```python
from build123d import *

# Parameters (mm, degrees)
EXTRUSION1_DEPTH      = 14
ESQUISSE3_R           = 7
EXTRUSION2_DEPTH      = 3.8
EXTRUSION2_DEPTH_BACK = 3.8
ESQUISSE4_R           = 2
EXTRUSION3_DEPTH      = 9


with BuildPart() as part:
    # Esquisse1 → Extrusion1 (new body)
    with BuildSketch(Plane.XY):
        with BuildLine():
            Line((8, 0), (6, 0))
            ThreePointArc((6, 0), (0, 6), (-6, 0))
            Line((-6, 0), (-8, 0))
            Line((-8, 0), (-8, 8))
            Line((-8, 8), (8, 8))
            Line((8, 8), (8, 0))
        make_face()
    extrude(amount=EXTRUSION1_DEPTH)

    # Esquisse3 → Extrusion2 (cut, two sides)
    with BuildSketch(Plane.XY.offset(7)) as extrusion2_sk:
        with Locations((0, -0.399862153)):
            Circle(ESQUISSE3_R)
    extrude(amount=EXTRUSION2_DEPTH, mode=Mode.SUBTRACT)
    extrude(extrusion2_sk.sketch, amount=-EXTRUSION2_DEPTH_BACK, mode=Mode.SUBTRACT)

    # Esquisse4 → Extrusion3 (cut, through all)
    with BuildSketch(Plane(origin=(0, 8, 0), x_dir=(1, 0, 0), z_dir=(0, 1, 0))):
        with Locations((-5, -7)):
            Circle(ESQUISSE4_R)
        with Locations((5, -7)):
            Circle(ESQUISSE4_R)
    extrude(amount=-EXTRUSION3_DEPTH, mode=Mode.SUBTRACT)


solid = part.part
```
Could you check a few things on this model? Use its own coordinates, in mm. A direction names the side the tool comes from. Coordinates: 2 decimals unless noted, no trailing zeros. Loops run counter-clockwise (first coordinate to the right, second up) from the corner with the lowest first, then second, coordinate; pieces in that order, holes last. Notation, with made-up numbers: M 55.5,-32.75 L 93.5,-32.75 A6 ccw 93.5,-28.75 Z; hole C 81,2.5 d9. An arc over 180 degrees is marked long. Put each result on its own line as item: value. Start each with the question number.
(1) Suppose I cut it at D-D on z = 7. Please give me the cut outline in (x, y), then the cut area to 3 significant figures.
(2) For faces 5 (the face through (0, 6, 12)), 6 (the face through (0.1, 6.6, 7.1)), which set-ups out of +Z, -Z, +X, -X, +Y, -Y let a thin tool reach every point of the face, with its end or its side?
(3) Suppose I cut it at C-C on y = 2.25. Please give me the cut outline in (x, z).
(4) Suppose I cut it at A-A on y = 7.5. Please give me the cut outline in (x, z), then the cut area to 3 significant figures.
(5) Will these pins go through, and if not, where does the flat tip stop? P1, Ø6.5, axis at x = 5, z = 7, coming from the -Y side; P2, Ø1.5, axis at x = -2, z = 4.5, coming from the -Y side.
(6) Suppose I cut it at B-B on x = 0. Please give me the cut outline in (y, z).
(7) Thinking about a two-plate mould opening in X: for faces 1 (the face through (-8, 4, 7)), 2 (the face through (-7, 6, 7)), 3 (the face through (0, 6.2, 10.8)), 4 (the face through (0, 7, 0)), which applies, pulls with the +X half, pulls with the -X half, needs draft (parallel to the pull), parting line crosses it, or undercut?
(8) I need wall thicknesses on line 1 (X direction, y = 5.5, z = 7); line 2 (Z direction, x = 5, y = 6); line 3 (Z direction, x = -5, y = 3.5). Which ranges of each line are inside material? Lowest first, please. Write a range as from..to.
Solutions:
1. outline: M -8,0 L -7,0 L -7,8 L -8,8 Z; M -3,5.92 A7 cw 3,5.92 L 3,8 L -3,8 Z; M 7,0 L 8,0 L 8,8 L 7,8 Z
1. area: 25.7 mm2
2. face 5: +Z, -Z, -Y
2. face 6: -Y
3. outline: M -8,0 L -5.56,0 L -5.56,3.2 L -6.48,3.2 L -6.48,5.65 A2 cw -6.48,8.35 L -6.48,10.8 L -5.56,10.8 L -5.56,14 L -8,14 Z; M 5.56,0 L 8,0 L 8,14 L 5.56,14 L 5.56,10.8 L 6.48,10.8 L 6.48,8.35 A2 cw 6.48,5.65 L 6.48,3.2 L 5.56,3.2 Z
4. outline: M -8,0 L 8,0 L 8,14 L -8,14 Z; hole C -5,7 d4; hole C 5,7 d4
4. area: 199 mm2
5. P1: stops at y = 0
5. P2: stops at y = 6.04
6. outline: M 6,0 L 8,0 L 8,14 L 6,14 L 6,10.8 L 6.6,10.8 L 6.6,3.2 L 6,3.2 Z
7. face 1: pulls with the -X half
7. face 2: undercut
7. face 3: undercut
7. face 4: needs draft
8. line 1: x = -8..-7, 7..8
8. line 2: z = 0..5, 9..14
8. line 3: z = 0..3.2, 10.8..14
